Geometry check sheet. Reference: the model listing, model coordinates, mm. Coordinates: 2 decimals unless noted, no trailing zeros. Loops run counter-clockwise (first coordinate to the right, second up) from the corner with the lowest first, then second, coordinate; pieces in that order, holes last.
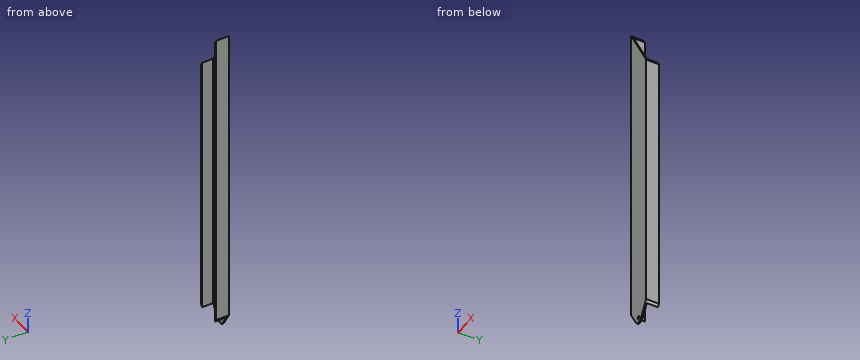
from build123d import *

# Parameters (mm, degrees)
BOSS_EXTRUDE1_DEPTH = 650.24
CUT_EXTRUDE1_DEPTH  = 652.231431674
SKETCH3_R           = 3.175
CUT_EXTRUDE2_DEPTH  = 652.231431674
FILLET1_R           = 7.62


with BuildPart() as part:
    # Sketch1 → Boss-Extrude1 (new body)
    with BuildSketch(Plane.XY):
        Polygon((-22.225, -9.525), (-22.225, 12.7), (-25.4, 12.7), (-25.4, -12.7), (25.4, -12.7), (25.4, 12.7), (22.225, 12.7), (22.225, -9.525), align=None)
    extrude(amount=BOSS_EXTRUDE1_DEPTH)

    # Sketch2 → Cut-Extrude1 (cut, through all)
    with BuildSketch(Plane.XZ.offset(12.7)):
        Polygon((-25.4, 650.24), (25.4, 562.251818976), (25.4, 650.24), align=None)
    extrude(amount=-CUT_EXTRUDE1_DEPTH, mode=Mode.SUBTRACT)

    # Sketch3 → Cut-Extrude2 (cut, through all)
    with BuildSketch(Plane(origin=(0, 12.7, 0), x_dir=(1, 0, 0), z_dir=(0, 1, 0))):
        with Locations(Location((0, -9.525, 0), (0, 0, 270))):
            Circle(SKETCH3_R)
        Polygon((-6.35, 0), (6.35, 0), (25.4, -32.995567884), (25.4, 20.936285304), (-25.4, 20.936285304), (-25.4, -32.995567884), align=None)
    extrude(amount=-CUT_EXTRUDE2_DEPTH, mode=Mode.SUBTRACT)

    # Fillet1
    fillet1_edges = [part.edges().sort_by_distance(p)[0] for p in [
        (6.35, -11.1125, 0),
        (-6.35, -11.1125, 0),
    ]]
    fillet(fillet1_edges, radius=FILLET1_R)


solid = part.part
1) Section check A-A on y = 7.5. Record the cut outline in (x, z) (3 decimals).
Data:
outline: (-25.4, 32.996) - (-22.225, 27.496) - (-22.225, 644.741) - (-25.4, 650.24) - close; (22.225, 27.496) - (25.4, 32.996) - (25.4, 562.252) - (22.225, 567.751) - close
2) Section check B-B on z = 255.5. Record the cut outline in (x, y) (3 decimals).
Data:
outline: (-25.4, -12.7) - (25.4, -12.7) - (25.4, 12.7) - (22.225, 12.7) - (22.225, -9.525) - (-22.225, -9.525) - (-22.225, 12.7) - (-25.4, 12.7) - close
3) Depth check by flat-ended pin: pin 1 (8 mm diameter, centred on x = 8, z = 310, fed in from +Y) (3 decimals); pin 2 (3 mm diameter, centred on x = 19.5, y = 3.5, fed in from +Z). Enter the tip coordinate at first touch or a pass-through.
Data:
pin 1: stops at y = -9.525
pin 2: passes through
4) Material ranges on probe 1 along X at (y, z) = (8, 118.5) (3 decimals); probe 2 along Y at (x, z) = (-17, 99.5) (3 decimals); probe 3 along Z at (x, y) = (21, -10), recorded low to high.
Data:
probe 1: x = -25.4 to -22.225, 22.225 to 25.4
probe 2: y = -12.7 to -9.525
probe 3: z = 25.37 to 569.87
